```python
from build123d import *

# Parameters (mm, degrees)
SKETCH1_W           = 155
SKETCH1_H           = 80
BOSS_EXTRUDE1_DEPTH = 2
SKETCH2_W           = 5
SKETCH2_H           = 7.8
BOSS_EXTRUDE2_DEPTH = 10
SKETCH3_R           = 1.45
CUT_EXTRUDE1_DEPTH  = 210
SKETCH4_R           = 1.45
CUT_EXTRUDE2_DEPTH  = 210


with BuildPart() as part:
    # Sketch1 → Boss-Extrude1 (new body)
    with BuildSketch(Plane(origin=(0, 0, 0), x_dir=(1, 0, 0), z_dir=(0, 1, 0))):
        with Locations((-77.5, 40)):
            Rectangle(SKETCH1_W, SKETCH1_H)
    extrude(amount=BOSS_EXTRUDE1_DEPTH)

    # Sketch2 → Boss-Extrude2 (add)
    with BuildSketch(Plane(origin=(0, 2, 0), x_dir=(1, 0, 0), z_dir=(0, 1, 0))):
        with Locations((-150.9, 74.5)):
            Rectangle(SKETCH2_W, SKETCH2_H)
        with Locations((-150.9, 5.5)):
            Rectangle(SKETCH2_W, SKETCH2_H)
        with Locations((-4.1, 74.5)):
            Rectangle(SKETCH2_W, SKETCH2_H)
        with Locations((-4.1, 5.5)):
            Rectangle(SKETCH2_W, SKETCH2_H)
    extrude(amount=BOSS_EXTRUDE2_DEPTH)

    # Sketch3 → Cut-Extrude1 (cut)
    with BuildSketch(Plane.ZY.offset(153.4)):
        with Locations((-5.5, 7)):
            Circle(SKETCH3_R)
    extrude(amount=-CUT_EXTRUDE1_DEPTH, mode=Mode.SUBTRACT)

    # Sketch4 → Cut-Extrude2 (cut)
    with BuildSketch(Plane(origin=(-1.6, 0, 0), x_dir=(0, 0, -1), z_dir=(1, 0, 0))):
        with Locations((74.5, 7)):
            Circle(SKETCH4_R)
    extrude(amount=-CUT_EXTRUDE2_DEPTH, mode=Mode.SUBTRACT)


solid = part.part
```
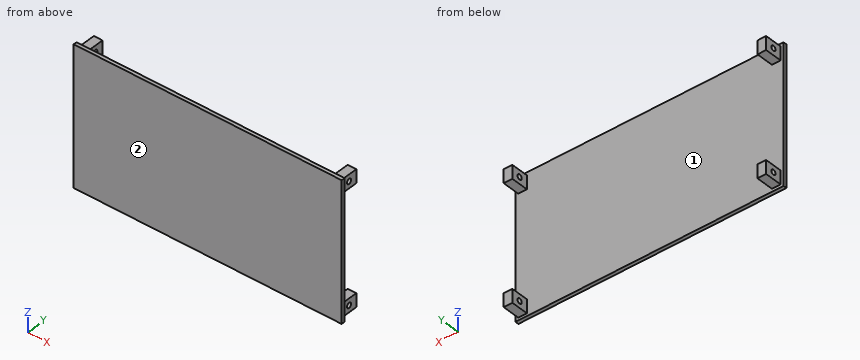
Design review of the part built by this model. Coordinates are the model's own, in mm. Face numbers are marked on the shaded views. Coordinates: 2 decimals unless noted, no trailing zeros. Write each loop counter-clockwise with the first axis right and the second up, starting at its lowest first coordinate (ties: lowest second). Pieces come first, ordered by that corner, then holes. Notation, with made-up numbers: M -8,50 L 1,50 A29 cw 1,86 Z; hole C 73,-11 d2. An arc over 180 degrees is marked long. Answer as a JSON object with one key per item and string values.
Item 1: Add section C-C, the plane x = -29.5. Give the boundary of the cut face in (y, z), and give its area (3 significant figures).
Outcome:
{"outline": "M 0,-80 L 2,-80 L 2,0 L 0,0 Z", "area": "160 mm²"}
Item 2: Add section D-D, the plane z = -31. Give the boundary of the cut face in (x, y).
Outcome:
{"outline": "M -155,0 L 0,0 L 0,2 L -155,2 Z"}
Item 3: Insertion check: pin 1 Ø1.5 at (x, y) = (-152, 5) entering from -Z; pin 2 Ø5.5 at (x, y) = (-150, 8.5) entering from +Z; pin 3 Ø6 at (y, z) = (7.5, -74) entering from +X; pin 4 Ø3 at (y, z) = (4, -29) entering from -X. Each pin has a flat end and moves straight along its axis. Give the tip position at first contact, or say it passes through.
Outcome:
{"pin 1": "z = -78.4", "pin 2": "z = -1.6", "pin 3": "x = -1.6", "pin 4": "through"}
Item 4: Wall thickness on probe 1 along Y at (x, z) = (-4.4, -5.5); probe 2 along Y at (x, z) = (-99, -41): over which ranges is each line inside the solid? List them lowest first.
Outcome:
{"probe 1": "0 to 5.55, 8.45 to 12", "probe 2": "0 to 2"}
Item 5: Add section B-B, the plane y = 7. State how many separate pieces and enclosed holes the cut face has, and give its area (3 significant figures).
Outcome:
{"separate pieces": "8", "enclosed holes": "0", "area": "98.0 mm²"}
Item 6: Add section A-A, the plane z = -5.5. Give the boundary of the cut face in (x, y), and give its area (3 significant figures).
Outcome:
{"outline": "M -155,0 L 0,0 L 0,2 L -1.6,2 L -1.6,5.55 L -6.6,5.55 L -6.6,2 L -148.4,2 L -148.4,5.55 L -153.4,5.55 L -153.4,2 L -155,2 Z; M -153.4,8.45 L -148.4,8.45 L -148.4,12 L -153.4,12 Z; M -6.6,8.45 L -1.6,8.45 L -1.6,12 L -6.6,12 Z", "area": "381 mm²"}
Item 7: Draft analysis for pull direction X (two halves, no side actions). For the marked faces 1 and 2, state which applies: pulls with the +X half, pulls with the -X half, needs draft (parallel to the pull), parting line crosses it, or undercut.
Outcome:
{"face 1": "undercut", "face 2": "needs draft"}
